Could you check a few things on this model? Use its own coordinates, in mm. Face numbers are marked on the shaded views. A direction names the side the tool comes from. Give positions to 0.01 mm unless a question says otherwise; leave off trailing zeros. Loops run counter-clockwise (first coordinate to the right, second up) from the corner with the lowest first, then second, coordinate; pieces in that order, holes last.
1. Thinking about a two-plate mould opening in Z: for the marked faces 1, 2 and 3, which applies, +Z half, -Z half, draft (parallel to the pull), parting line (faces both ways), or undercut?
2. I need wall thicknesses on line 1 along Y through (x, z) = (0, 1); line 2 along Y through (x, z) = (6, 26); line 3 along Y through (x, z) = (12, 3). Which ranges of each line are inside material? Lowest first, please.
3. Imagine slicing it at A-A (y = 0). List the corners of the cut face in (x, z) for me.
4. For the marked faces 4, 5 and 6, which set-ups out of +Z, -Z, +X, -X, +Y, -Y let a thin tool reach every point of the face, with its end or its side?
5. Imagine slicing it at C-C (x = 20.5). List the corners of the cut face in (y, z) for me, plus the area to 3 significant figures.
6. For P1, Ø6, axis at x = -12.5, y = -24, coming from the +Z side; P2, Ø2, axis at x = 23, z = 4.5, coming from the +Y side; P3, Ø3, axis at x = 12, z = 11.5, coming from the +Y side, each with a flat end and sliding along its axis, tell me the tip position at first contact or that it passes through.
7. Imagine slicing it at D-D (z = 39.4). List the corners of the cut face in (x, y) for me.
8. Imagine slicing it at B-B (z = 25). List the corners of the cut face in (x, y) for me.
```python
from build123d import *

# Parameters (mm, degrees)
BOSS_EXTRUDE1_DEPTH                                 = 8
CUT_EXTRUDE1_REACH                                  = 5
SKETCH4_W                                           = 55.8
SKETCH4_H                                           = 37.4
BOSS_EXTRUDE2_DEPTH                                 = 37.4
BOSS_EXTRUDE3_DEPTH                                 = 3
CUT_EXTRUDE2_DEPTH                                  = 3
CUT_EXTRUDE3_DEPTH                                  = 3
CSK_FOR_8_FLAT_HEAD_MACHINE_SCREW_100_D             = 4.5
CSK_FOR_8_FLAT_HEAD_MACHINE_SCREW_100_DEPTH         = 8
CSK_FOR_8_FLAT_HEAD_MACHINE_SCREW_100_CSINK_D       = 9.4
CSK_FOR_8_FLAT_HEAD_MACHINE_SCREW_100_CSINK_ANGLE   = 90
F_4_CLEARANCE_HOLE1_D                               = 3.3
F_4_CLEARANCE_HOLE1_DEPTH                           = 6
CBORE_FOR_8_BINDING_HEAD_MACHINE_SCREW1_D           = 4.5
CBORE_FOR_8_BINDING_HEAD_MACHINE_SCREW1_DEPTH       = 8
CBORE_FOR_8_BINDING_HEAD_MACHINE_SCREW1_CBORE_D     = 7.5
CBORE_FOR_8_BINDING_HEAD_MACHINE_SCREW1_CBORE_DEPTH = 3
FILLET1_R                                           = 6.35
M3X0_5_TAPPED_HOLE1_D                               = 2.5
M3X0_5_TAPPED_HOLE1_DEPTH                           = 4
M3X0_5_TAPPED_HOLE1_TIP                             = 0.751075774
FILLET2_R                                           = 6.35


with BuildPart() as part:
    # Sketch1 → Boss-Extrude1 (new body)
    with BuildSketch(Plane.XY.offset(8)):
        with BuildLine():
            Line((-23.45868709, 18.7), (-23.45868709, -18.7))
            ThreePointArc((-23.45868709, -18.7), (0, -30), (23.45868709, -18.7))
            Line((23.45868709, -18.7), (35.34131291, -18.7))
            Line((35.34131291, -18.7), (35.34131291, 18.7))
            Line((35.34131291, 18.7), (23.45868709, 18.7))
            ThreePointArc((23.45868709, 18.7), (0, 30), (-23.45868709, 18.7))
        make_face()
    extrude(amount=-BOSS_EXTRUDE1_DEPTH)

    # Sketch3 → Cut-Extrude1 (cut, up to next)
    with BuildSketch(Plane(origin=(-20.45868709, 0, 0), x_dir=(0, 0, -1), z_dir=(1, 0, 0)), mode=Mode.PRIVATE) as cut_extrude1_sk1:
        with BuildLine():
            Line((-8, 18.7), (-8, -18.7))
            ThreePointArc((-8, -18.7), (-0.254206384, 0), (-8, 18.7))
        make_face()
    cut_extrude1_tool1 = extrude(cut_extrude1_sk1.sketch, amount=-CUT_EXTRUDE1_REACH, mode=Mode.PRIVATE) & part.part
    add(cut_extrude1_tool1.solids().sort_by_distance((-20.458687, 0, 4.859168))[0], mode=Mode.SUBTRACT)

    # Sketch4 → Boss-Extrude2 (add)
    with BuildSketch(Plane.XY.offset(8)):
        with Locations((7.44131291, 0)):
            Rectangle(SKETCH4_W, SKETCH4_H)
    extrude(amount=BOSS_EXTRUDE2_DEPTH)

    # Sketch5 → Boss-Extrude3 (add)
    with BuildSketch(Plane.ZY.offset(20.45868709)):
        with BuildLine():
            Line((21.171890016, 18.7), (45.4, 18.7))
            Line((45.4, 18.7), (45.4, -18.7))
            Line((45.4, -18.7), (21.171890016, -18.7))
            ThreePointArc((21.171890016, -18.7), (7.2, 0), (21.171890016, 18.7))
        make_face()
    extrude(amount=BOSS_EXTRUDE3_DEPTH)

    # Sketch6 → Cut-Extrude2 (cut)
    with BuildSketch(Plane.ZY.offset(23.45868709)):
        with BuildLine():
            Line((45.4, -18.7), (45.4, -5.528109984))
            ThreePointArc((45.4, -5.528109984), (40.488582233, -13.788582233), (32.228109984, -18.7))
            Line((32.228109984, -18.7), (45.4, -18.7))
        make_face()
    extrude(amount=-CUT_EXTRUDE2_DEPTH, mode=Mode.SUBTRACT)

    # Sketch7 → Cut-Extrude3 (cut)
    with BuildSketch(Plane.ZY.offset(23.45868709)):
        with BuildLine():
            Line((45.4, 18.7), (32.228109984, 18.7))
            ThreePointArc((32.228109984, 18.7), (40.488582233, 13.788582233), (45.4, 5.528109984))
            Line((45.4, 5.528109984), (45.4, 18.7))
        make_face()
    extrude(amount=-CUT_EXTRUDE3_DEPTH, mode=Mode.SUBTRACT)

    # Sketch8 → Cut-Revolve1 (revolve, cut)
    with BuildSketch(Plane.XY.offset(26.7)):
        Polygon((-23.45868709, 15.86865), (-23.45868709, 0), (35.34131291, 0), (35.34131291, 15.86865), (9.94131291, 15.86865), (9.94131291, 13.5), (1.94131291, 13.5), (1.94131291, 15.86865), align=None)
    revolve(axis=Axis((-23.45868709, 0, 26.7), (1, 0, 0)), mode=Mode.SUBTRACT)

    # CSK for #8 Flat Head Machine Screw (100)1
    with Locations(Plane.XY.offset(8)):
        with Locations((0, 25.5), (0, -25.5)):
            CounterSinkHole(CSK_FOR_8_FLAT_HEAD_MACHINE_SCREW_100_D / 2, CSK_FOR_8_FLAT_HEAD_MACHINE_SCREW_100_CSINK_D / 2, depth=CSK_FOR_8_FLAT_HEAD_MACHINE_SCREW_100_DEPTH, counter_sink_angle=CSK_FOR_8_FLAT_HEAD_MACHINE_SCREW_100_CSINK_ANGLE)

    # #4 Clearance Hole1
    with Locations(Plane(origin=(0, -18.7, 0), x_dir=(-1, 0, 0), z_dir=(0, -1, 0))):
        with Locations((12.45868709, -39.4), (-29.44131291, -39.4), (-29.44131291, -5.9)):
            Hole(F_4_CLEARANCE_HOLE1_D / 2, depth=F_4_CLEARANCE_HOLE1_DEPTH)

    # CBORE for #8 Binding Head Machine Screw1
    with Locations(Plane.XY.offset(8)):
        with Locations((12, 22.95), (-12, 22.95), (-12, -22.95), (12, -22.95)):
            CounterBoreHole(CBORE_FOR_8_BINDING_HEAD_MACHINE_SCREW1_D / 2, CBORE_FOR_8_BINDING_HEAD_MACHINE_SCREW1_CBORE_D / 2, CBORE_FOR_8_BINDING_HEAD_MACHINE_SCREW1_CBORE_DEPTH, depth=CBORE_FOR_8_BINDING_HEAD_MACHINE_SCREW1_DEPTH)

    # Fillet1
    fillet1_edges = [part.edges().sort_by_distance(p)[0] for p in [
        (23.45868709, 18.7, 4),
    ]]
    fillet(fillet1_edges, radius=FILLET1_R)

    # M3x0.5 Tapped Hole1
    with Locations(Plane(origin=(1.04131291, 8.07366885, 45.4), x_dir=(1, 0, 0), z_dir=(0, 0, 1))):
        with Locations((0, 0), (10.150400418, -22.272670952)):
            Hole(M3X0_5_TAPPED_HOLE1_D / 2, depth=M3X0_5_TAPPED_HOLE1_DEPTH)
            with Locations((0, 0, -(M3X0_5_TAPPED_HOLE1_DEPTH + M3X0_5_TAPPED_HOLE1_TIP / 2))):  # 118° drill point
                Cone(0, M3X0_5_TAPPED_HOLE1_D / 2, M3X0_5_TAPPED_HOLE1_TIP, mode=Mode.SUBTRACT)

    # Fillet2
    fillet2_edges = [part.edges().sort_by_distance(p)[0] for p in [
        (23.45868709, -18.7, 4),
    ]]
    fillet(fillet2_edges, radius=FILLET2_R)


solid = part.part
```
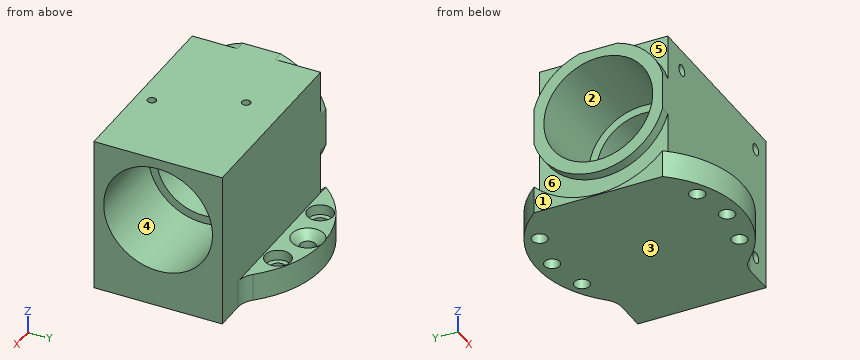
Derived:
1. face 1: draft
1. face 2: undercut
1. face 3: -Z half
2. line 1: y = -30 to -27.75, -23.25 to 23.25, 27.75 to 30
2. line 2: y = -18.7 to -13.48, 13.48 to 18.7
2. line 3: y = -27.5 to -25.2, -20.7 to 20.7, 25.2 to 27.5
3. outline: (-23.46, 0) - (35.34, 0) - (35.34, 10.83) - (9.94, 10.83) - (9.94, 13.2) - (1.94, 13.2) - (1.94, 10.83) - (-23.46, 10.83) - (-23.46, 7.2) - (-20.46, 7.2) - (-20.46, 0.25) - (-23.46, 0.25) - close; (-23.46, 42.57) - (1.94, 42.57) - (1.94, 40.2) - (9.94, 40.2) - (9.94, 42.57) - (35.34, 42.57) - (35.34, 45.4) - (-23.46, 45.4) - close
4. face 4: +X
4. face 5: +Z, -X, -Y
4. face 6: -X
5. outline: (-21.9, 0) - (21.9, 0) - (21.9, 8) - (18.7, 8) - (18.7, 45.4) - (-18.7, 45.4) - (-18.7, 8) - (-21.9, 8) - close; hole circle Ø31.74 at (0, 26.7)
5. area: 958 mm2
6. P1: stops at z = 8
6. P2: stops at y = 20.42
6. P3: stops at y = 18.7
7. outline: (-23.46, -14.8) - (-20.46, -14.8) - (-20.46, -18.7) - (-14.11, -18.7) - (-14.11, -12.7) - (-10.81, -12.7) - (-10.81, -18.7) - (27.79, -18.7) - (27.79, -12.7) - (31.09, -12.7) - (31.09, -18.7) - (35.34, -18.7) - (35.34, -9.51) - (9.94, -9.51) - (9.94, -4.58) - (1.94, -4.58) - (1.94, -9.51) - (-23.46, -9.51) - close; (-23.46, 9.51) - (1.94, 9.51) - (1.94, 4.58) - (9.94, 4.58) - (9.94, 9.51) - (35.34, 9.51) - (35.34, 18.7) - (-20.46, 18.7) - (-20.46, 14.8) - (-23.46, 14.8) - close
8. outline: (-23.46, -18.7) - (35.34, -18.7) - (35.34, -15.78) - (9.94, -15.78) - (9.94, -13.39) - (1.94, -13.39) - (1.94, -15.78) - (-23.46, -15.78) - close; (-23.46, 15.78) - (1.94, 15.78) - (1.94, 13.39) - (9.94, 13.39) - (9.94, 15.78) - (35.34, 15.78) - (35.34, 18.7) - (-23.46, 18.7) - close
